Can you work these out from the model? Positions are in its coordinate system, mm. Round coordinates to 2 decimals unless told otherwise and drop trailing zeros. Write each loop counter-clockwise with the first axis right and the second up, starting at its lowest first coordinate (ties: lowest second). Pieces come first, ordered by that corner, then holes. Notation, with made-up numbers: (-38.5, 14) -> (-10.5, 14) arc R3 ccw to (-10.5, 18) -> close; hole circle Ø5 at (63, 14). An arc over 180 degrees is marked (long way). Use CSV: the item, a comma, the result in double quotes.
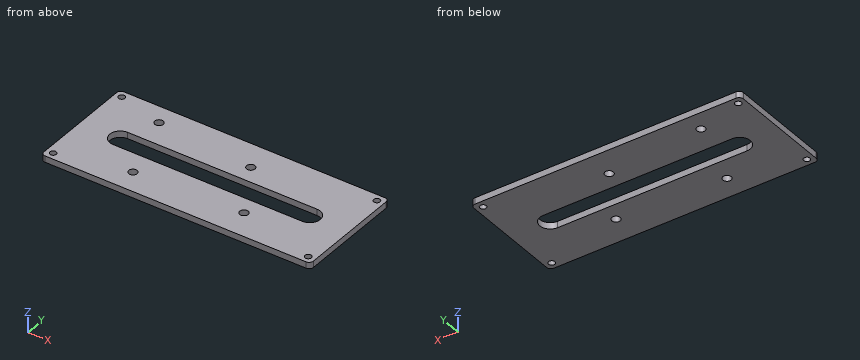
```python
from build123d import *

# Parameters (mm, degrees)
ESQUISSE1_W             = 128
ESQUISSE1_H             = 53
BOSS_EXTRU_1_DEPTH      = 3
ESQUISSE2_R             = 2
ENL_V_MAT_EXTRU_1_DEPTH = 3
ENL_V_MAT_EXTRU_2_DEPTH = 3
ESQUISSE5_R             = 1.5
ENL_V_MAT_EXTRU_3_DEPTH = 3
CONG_1_R                = 2


with BuildPart() as part:
    # Esquisse1 → Boss.-Extru.1 (new body)
    with BuildSketch(Plane.XY):
        Rectangle(ESQUISSE1_W, ESQUISSE1_H)
    extrude(amount=BOSS_EXTRU_1_DEPTH)

    # Esquisse2 → Enlèv. mat.-Extru.1 (cut)
    with BuildSketch(Plane.XY.offset(3)):
        with Locations((-38.82, 17.35)):
            Circle(ESQUISSE2_R)
        with Locations((7.66, 13.27)):
            Circle(ESQUISSE2_R)
        with Locations((-27.89, -15.71)):
            Circle(ESQUISSE2_R)
        with Locations((23.18, -13.35)):
            Circle(ESQUISSE2_R)
    extrude(amount=-ENL_V_MAT_EXTRU_1_DEPTH, mode=Mode.SUBTRACT)

    # Esquisse3 → Enlèv. mat.-Extru.2 (cut)
    with BuildSketch(Plane.XY.offset(3)):
        with BuildLine():
            Line((-45.000000383, 5), (45.000000383, 5))
            ThreePointArc((45.000000383, 5), (50.000000383, 0), (45.000000383, -5))
            Line((45.000000383, -5), (-44.999999617, -5))
            ThreePointArc((-44.999999617, -5), (-49.999999617, -3.83e-07), (-45.000000383, 5))
        make_face()
    extrude(amount=-ENL_V_MAT_EXTRU_2_DEPTH, mode=Mode.SUBTRACT)

    # Esquisse5 → Enlèv. mat.-Extru.3 (cut)
    with BuildSketch(Plane.XY.offset(3)):
        with Locations((-60.62, 23.12)):
            Circle(ESQUISSE5_R)
        with Locations((60.62, 23.12)):
            Circle(ESQUISSE5_R)
        with Locations((-60.62, -23.12)):
            Circle(ESQUISSE5_R)
        with Locations((60.62, -23.12)):
            Circle(ESQUISSE5_R)
    extrude(amount=-ENL_V_MAT_EXTRU_3_DEPTH, mode=Mode.SUBTRACT)

    # Congé1
    cong_1_edges = [part.edges().sort_by_distance(p)[0] for p in [
        (-64, 26.5, 1.5),
        (64, 26.5, 1.5),
        (64, -26.5, 1.5),
        (-64, -26.5, 1.5),
    ]]
    fillet(cong_1_edges, radius=CONG_1_R)


solid = part.part
```
Q1. Suppose I cut it at A-A (y = 0). Write out the boundary of the cut face in (x, z), and give its area (3 significant figures).
Resolved:
outline,"(-64, 0) -> (-50, 0) -> (-50, 3) -> (-64, 3) -> close; (50, 0) -> (64, 0) -> (64, 3) -> (50, 3) -> close"
area,"84.0 mm^2"
Q2. Suppose I cut it at B-B (x = 60.62). Write out the boundary of the cut face in (y, z).
Resolved:
outline,"(-26.5, 0) -> (-24.62, 0) -> (-24.62, 3) -> (-26.5, 3) -> close; (-21.62, 0) -> (21.62, 0) -> (21.62, 3) -> (-21.62, 3) -> close; (24.62, 0) -> (26.5, 0) -> (26.5, 3) -> (24.62, 3) -> close"
Q3. Suppose I cut it at C-C (z = 1.8). Count the separate pieces of the cut face and the enclosed holes in it, and give its area (3 significant figures).
Resolved:
separate pieces,"1"
enclosed holes,"9"
area,"5,720 mm^2"
Q4. Please list where these lines run through material, in increasing order: probe 1 along Y at (x, z) = (-38.82, 1.8); probe 2 along Y at (x, z) = (23.18, 2); probe 3 along Y at (x, z) = (-20, 2.1).
Resolved:
probe 1,"y = -26.5 to -5, 5 to 15.35, 19.35 to 26.5"
probe 2,"y = -26.5 to -15.35, -11.35 to -5, 5 to 26.5"
probe 3,"y = -26.5 to -5, 5 to 26.5"
Q5. Suppose I cut it at D-D (x = -48). Write out the boundary of the cut face in (y, z), and give its area (3 significant figures).
Resolved:
outline,"(-26.5, 0) -> (-4, 0) -> (-4, 3) -> (-26.5, 3) -> close; (4, 0) -> (26.5, 0) -> (26.5, 3) -> (4, 3) -> close"
area,"135 mm^2"
Q6. Will this pin go through, and if not, where does the flat tip stop? P1, Ø3.5, axis at x = -27.89, y = -15.71, coming from the +Z side.
Resolved:
P1,"passes through"
